```python
from build123d import *

# Parameters (mm, degrees)
F0_R      = 1.9812
F0_W      = 73.1012
F0_H      = 55.499
F1_DEPTH  = 2.032
F2_W      = 99.06
F2_H      = 72.9742
F3_DEPTH  = 1.905
F4_W      = 99.06
F4_H      = 72.9742
F4_W_2    = 96.774
F4_H_2    = 66.8528
F5_DEPTH  = 6.35
F6_R      = 2.7051
F6_R_2    = 1.016
F7_DEPTH  = 17.78
F8_R      = 2.7051
F8_R_2    = 1.016
F9_DEPTH  = 4.572
F12_DEPTH = 3.175
F15_DEPTH = 3.175


with BuildPart() as f1:
    # F0 (on Top) → F1 (new body)
    with BuildSketch(Plane.XY):
        with BuildLine():
            Line((56.515, 46.99), (-56.515, 46.99))
            ThreePointArc((-56.515, 46.99), (-58.760064, 46.060064), (-59.69, 43.815))
            Line((-59.69, 43.815), (-59.69, -43.815))
            ThreePointArc((-59.69, -43.815), (-58.760064, -46.060064), (-56.515, -46.99))
            Line((-56.515, -46.99), (56.515, -46.99))
            ThreePointArc((56.515, -46.99), (58.760064, -46.060064), (59.69, -43.815))
            Line((59.69, -43.815), (59.69, 43.815))
            ThreePointArc((59.69, 43.815), (58.760064, 46.060064), (56.515, 46.99))
        make_face()
        with Locations((-53.34, -40.64)):
            Circle(F0_R, mode=Mode.SUBTRACT)
        with Locations((53.34, -40.64)):
            Circle(F0_R, mode=Mode.SUBTRACT)
        Rectangle(F0_W, F0_H, mode=Mode.SUBTRACT)
        with Locations((-53.34, 40.64)):
            Circle(F0_R, mode=Mode.SUBTRACT)
        with Locations((53.34, 40.64)):
            Circle(F0_R, mode=Mode.SUBTRACT)
    extrude(amount=F1_DEPTH)

    # F2 (on face) → F3 (join)
    with BuildSketch(Plane.XY.offset(2.032)):
        Rectangle(F2_W, F2_H)
        Polygon((38.6842, -32.1818), (-38.6842, -32.1818), (-38.6842, 32.1818), (-25.415266, 32.1818), (-25.415266, 33.4518), (25.384734, 33.4518), (25.384734, 32.1818), (38.6842, 32.1818), align=None, mode=Mode.SUBTRACT)
    extrude(amount=F3_DEPTH)

    # F4 (on face) → F5 (join)
    with BuildSketch(Plane.XY.offset(3.937)):
        Rectangle(F4_W, F4_H)
        Rectangle(F4_W_2, F4_H_2, mode=Mode.SUBTRACT)
    extrude(amount=F5_DEPTH)

    # F6 (on face) → F7 (join)
    with BuildSketch(Plane.XY.offset(3.937)):
        with Locations((-42.799, 27.8511)):
            Circle(F6_R)
        with Locations((-42.799, 27.8511)):
            Circle(F6_R_2, mode=Mode.SUBTRACT)
        with Locations((-42.799, -27.8511)):
            Circle(F6_R)
        with Locations((-42.799, -27.8511)):
            Circle(F6_R_2, mode=Mode.SUBTRACT)
        with Locations((42.799, -27.8511)):
            Circle(F6_R)
        with Locations((42.799, -27.8511)):
            Circle(F6_R_2, mode=Mode.SUBTRACT)
        with Locations((42.799, 27.8511)):
            Circle(F6_R)
        with Locations((42.799, 27.8511)):
            Circle(F6_R_2, mode=Mode.SUBTRACT)
    extrude(amount=F7_DEPTH)

    # F8 (on face) → F9 (join)
    with BuildSketch(Plane.XY.offset(3.937)):
        with Locations((-42.799, 19.05)):
            Circle(F8_R)
        with Locations((-42.799, 19.05)):
            Circle(F8_R_2, mode=Mode.SUBTRACT)
        with Locations((-42.799, -19.05)):
            Circle(F8_R)
        with Locations((-42.799, -19.05)):
            Circle(F8_R_2, mode=Mode.SUBTRACT)
        with Locations((42.799, 19.05)):
            Circle(F8_R)
        with Locations((42.799, 19.05)):
            Circle(F8_R_2, mode=Mode.SUBTRACT)
        with Locations((42.799, -19.05)):
            Circle(F8_R)
        with Locations((42.799, -19.05)):
            Circle(F8_R_2, mode=Mode.SUBTRACT)
    extrude(amount=F9_DEPTH)

    # F11 (on offset) → F12 (join, symmetric)
    with BuildSketch(Plane.YZ.offset(-25.4)):
        with BuildLine():
            Line((-34.9504, 10.287), (-33.4264, 10.287))
            Line((-33.4264, 10.287), (-33.4264, 24.721494))
            ThreePointArc((-33.4264, 24.721494), (-33.636293, 24.971636), (-33.919082, 24.808368))
            Line((-33.919082, 24.808368), (-35.763301, 19.741417))
            Line((-35.763301, 19.741417), (-35.763301, 18.830367))
            Line((-35.763301, 18.830367), (-35.4584, 18.467))
            Line((-35.4584, 18.467), (-34.9504, 18.467))
            Line((-34.9504, 18.467), (-34.9504, 10.287))
        make_face()
        with BuildLine():
            Line((33.4264, 24.721494), (33.4264, 10.287))
            Line((33.4264, 10.287), (34.9504, 10.287))
            Line((34.9504, 10.287), (34.9504, 18.467))
            Line((34.9504, 18.467), (35.4584, 18.467))
            Line((35.4584, 18.467), (35.763301, 18.830367))
            Line((35.763301, 18.830367), (35.763301, 19.741417))
            Line((35.763301, 19.741417), (33.919082, 24.808368))
            ThreePointArc((33.919082, 24.808368), (33.636293, 24.971636), (33.4264, 24.721494))
        make_face()
    extrude(amount=F12_DEPTH, both=True)

    # F14 (on offset) → F15 (join, symmetric)
    with BuildSketch(Plane.YZ.offset(25.4)):
        with BuildLine():
            ThreePointArc((33.919082, 24.808368), (33.636293, 24.971636), (33.4264, 24.721494))
            Line((33.4264, 24.721494), (33.4264, 10.287))
            Line((33.4264, 10.287), (34.9504, 10.287))
            Line((34.9504, 10.287), (34.9504, 18.467))
            Line((34.9504, 18.467), (35.4584, 18.467))
            Line((35.4584, 18.467), (35.763301, 18.830367))
            Line((35.763301, 18.830367), (35.763301, 19.741417))
            Line((35.763301, 19.741417), (33.919082, 24.808368))
        make_face()
    extrude(amount=F15_DEPTH, both=True)


solid = f1.part
```
Model file for the job. Use its own axes, mm. A direction names the side the tool comes from. Coordinates: 2 decimals unless noted, no trailing zeros. Order: outer loops, then holes, each group sorted by start corner. A loop starts at its lowest first (then second) coordinate and runs counter-clockwise, first axis right, second up. Notation, with made-up numbers: M 82.5,14.25 L 113.5,14.25 A24 cw 113.5,29.25 Z; hole C -27,75 d8. An arc over 180 degrees is marked long. Answer as CSV lines item,"result".
(1) Flat gauge pins, fed straight in: pin 1 (3 mm diameter, centred on x = 43.5, z = 7.5, fed in from +Y); pin 2 (1 mm diameter, centred on x = -25, z = 19, fed in from +Y); pin 3 (1 mm diameter, centred on x = -43, y = -28, fed in from +Z); pin 4 (8 mm diameter, centred on x = -36, z = 17.5, fed in from +Y). Where does each tip first touch, or does it go through?
Geometry says:
pin 1,"stops at y = 36.49"
pin 2,"stops at y = 35.76"
pin 3,"stops at z = 3.94"
pin 4,"passes through"
(2) Band-saw the part on C-C, the plane y = -40.64. List the corners of the cut face in (x, z).
Geometry says:
outline,"M -59.69,0 L -55.32,0 L -55.32,2.03 L -59.69,2.03 Z; M -51.36,0 L 51.36,0 L 51.36,2.03 L -51.36,2.03 Z; M 55.32,0 L 59.69,0 L 59.69,2.03 L 55.32,2.03 Z"
(3) Band-saw the part on B-B, the plane z = 6.75. State how many separate pieces and enclosed holes the cut face has, then the cut area to 3 significant figures.
Geometry says:
separate pieces,"9"
enclosed holes,"9"
area,"917 mm2"
(4) 3-axis set-ups, long thin cutter, end or side, ignore diameter. For faces 1 (the cylindrical face through (58.78, 46.04, 1)), 2 (the flat face through (-22.225, 34, 18)), 3 (the flat face through (44, 28, 21.717)), 4 (the flat face through (-40, 0, 3.937)), 5 (the flat face through (49.53, -1, 6)): which of +Z, -Z, +X, -X, +Y, -Y reach the whole face in a straight line?
Geometry says:
face 1,"+Z, -Z, +X, +Y"
face 2,"+Z, +Y, -Y"
face 3,"+Z, +X, -X, +Y, -Y"
face 4,"+Z"
face 5,"+Z, +X, +Y, -Y"
(5) Wall check: line 1 along Y through (x, z) = (-53.34, 0.65); line 2 along X through (y, z) = (-11, 6.5); line 3 along Y through (x, z) = (5, 2.25). Give the ranges that are in metal, low to high.
Geometry says:
line 1,"y = -46.99 to -42.62, -38.66 to 38.66, 42.62 to 46.99"
line 2,"x = -49.53 to -48.39, 48.39 to 49.53"
line 3,"y = -36.49 to -32.18, 33.45 to 36.49"
(6) Pull direction Y, two halves, no side cores. Call faces 6 (the cylindrical face through (58.74, -46.08, 1)), 7 (the flat face through (44, 19, 8.509)), 8 (the flat face through (-43, -29, 21.717)): +Y half, -Y half, draft (parallel to the pull), parting line (faces both ways), or undercut.
Geometry says:
face 6,"-Y half"
face 7,"undercut"
face 8,"draft"
(7) Band-saw the part on A-A, the plane x = 53.34. List the corners of the cut face in (y, z).
Geometry says:
outline,"M -46.99,0 L -42.62,0 L -42.62,2.03 L -46.99,2.03 Z; M -38.66,0 L 38.66,0 L 38.66,2.03 L -38.66,2.03 Z; M 42.62,0 L 46.99,0 L 46.99,2.03 L 42.62,2.03 Z"
